from build123d import *

# Parameters (mm, degrees)
BOSS_EXTRUDE1_DEPTH = 25
SKETCH2_W           = 50
SKETCH2_H           = 35
SKETCH2_H_2         = 7.5
BOSS_EXTRUDE2_DEPTH = 100
SKETCH3_W           = 5
SKETCH3_H           = 7.5
BOSS_EXTRUDE3_DEPTH = 75
SKETCH4_W           = 10
SKETCH4_H           = 40
BOSS_EXTRUDE4_DEPTH = 7.5
CUT_EXTRUDE1_REACH  = 122.52
SKETCH5_W           = 30
SKETCH5_H           = 15
SKETCH7_W           = 42
SKETCH7_H           = 92
SKETCH7_W_2         = 38
SKETCH7_H_2         = 88
CUT_EXTRUDE2_DEPTH  = 15


with BuildPart() as part:
    # Sketch1 → Boss-Extrude1 (new, symmetric)
    with BuildSketch(Plane.XY):
        Polygon((0, 0), (45, 0), (0, 25), (-5, 25), (-5, 0), align=None)
    extrude(amount=BOSS_EXTRUDE1_DEPTH, both=True)

    # Sketch2 → Boss-Extrude2 (add)
    with BuildSketch(Plane(origin=(0, 0, 0), x_dir=(1, 0, 0), z_dir=(0, 1, 0))):
        with Locations((20, -7.5)):
            Rectangle(SKETCH2_W, SKETCH2_H)
        with Locations((20, 21.25)):
            Rectangle(SKETCH2_W, SKETCH2_H_2)
    extrude(amount=BOSS_EXTRUDE2_DEPTH)

    # Sketch3 → Boss-Extrude3 (add)
    with BuildSketch(Plane(origin=(0, 25, 0), x_dir=(1, 0, 0), z_dir=(0, 1, 0))):
        with Locations((-2.5, 13.75)):
            Rectangle(SKETCH3_W, SKETCH3_H)
    extrude(amount=BOSS_EXTRUDE3_DEPTH)

    # Sketch4 → Boss-Extrude4 (add)
    with BuildSketch(Plane.XY.offset(-17.5)):
        with Locations((40, 80)):
            Rectangle(SKETCH4_W, SKETCH4_H)
    extrude(amount=BOSS_EXTRUDE4_DEPTH)

    # Sketch5 → Cut-Extrude1 (cut, up to next)
    with BuildSketch(Plane.XY.offset(25), mode=Mode.PRIVATE) as cut_extrude1_sk1:
        with Locations((17.5, 77.5)):
            Rectangle(SKETCH5_W, SKETCH5_H)
    cut_extrude1_tool1 = extrude(cut_extrude1_sk1.sketch, amount=-CUT_EXTRUDE1_REACH, mode=Mode.PRIVATE) & part.part
    add(cut_extrude1_tool1.solids().sort_by_distance((17.5, 77.5, 25))[0], mode=Mode.SUBTRACT)

    # Sketch7 → Cut-Extrude2 (cut)
    with BuildSketch(Plane.XY.offset(25)):
        with Locations((20, 50)):
            Rectangle(SKETCH7_W, SKETCH7_H)
        with Locations((20, 50)):
            Rectangle(SKETCH7_W_2, SKETCH7_H_2, mode=Mode.SUBTRACT)
    extrude(amount=-CUT_EXTRUDE2_DEPTH, mode=Mode.SUBTRACT)


solid = part.part
CAD build for the part. Positions are in the model's coordinates, mm. A direction names the side the tool comes from. Give positions to 0.01 mm unless a question says otherwise; leave off trailing zeros. Loops run counter-clockwise (first coordinate to the right, second up) from the corner with the lowest first, then second, coordinate; pieces in that order, holes last. Notation, with made-up numbers: M -20,-19 L -6,-19 A8 ccw -6,-15 Z; hole C 64,-2 d4. An arc over 180 degrees is marked long. Answer in a Markdown table with one row per item. Add a question column.
Item 1: Probe probe 1 along X at (y, z) = (47.5, 12.5); probe 2 along Y at (x, z) = (18, 20); probe 3 along X at (y, z) = (83.5, 21). List the from-to ranges inside material, lowest first.
Item 2: Band-saw the part on B-B on y = 64. Give the cut face in (x, z).
Item 3: Drop flat-ended pins along their axis: P1, Ø1.5, axis at x = 7, z = -11.5, coming from the +Y side; P2, Ø2, axis at x = 8, y = 72, coming from the +Z side. Give the stop position or say it passes through.
Item 4: Band-saw the part on C-C on x = 31. Give the cut face in (y, z).
Item 5: Band-saw the part on D-D on z = -13. Give the cut face in (x, y).
Item 6: Mould opens along X. For faces 5 (the face through (40, 60, -14)), 6 (the face through (20, 4, 18)), 7 (the face through (-5, 49, 0)) say: +X half, -X half, draft (parallel to the pull), parting line (faces both ways), or undercut.
Item 7: Band-saw the part on A-A on z = 6. Give the cut face in (x, y).
Item 8: Tool access for faces 1 (the face through (20, 94, 18)), 2 (the face through (0, 62, -14)), 3 (the face through (22, 49, -17.5)), 4 (the face through (20, 51, -25)): list every direction of +Z, -Z, +X, -X, +Y, -Y with a clear straight run to the whole face (end or side of a thin tool).
Reply:
| question | item | result |
|---|---|---|
| 1 | probe 1 | x = -5 to -1, 1 to 39, 41 to 45 |
| 1 | probe 2 | y = 0 to 4, 6 to 70, 85 to 94, 96 to 100 |
| 1 | probe 3 | x = -5 to -1, 1 to 2.5, 32.5 to 39, 41 to 45 |
| 2 | outline | M -5,-25 L 45,-25 L 45,25 L 41,25 L 41,10 L 39,10 L 39,25 L 1,25 L 1,10 L -1,10 L -1,25 L -5,25 Z; hole M 0,-17.5 L 35,-17.5 L 35,-10 L 0,-10 Z |
| 3 | P1 | stops at y = 21.53 |
| 3 | P2 | stops at z = -17.5 |
| 4 | outline | M 0,-25 L 100,-25 L 100,-17.5 L 7.78,-17.5 L 7.78,-10 L 70,-10 L 70,25 L 6,25 L 6,10 L 4,10 L 4,25 L 0,25 Z; M 85,-10 L 100,-10 L 100,25 L 96,25 L 96,10 L 94,10 L 94,25 L 85,25 Z |
| 5 | outline | M -5,0 L 45,0 L 0,25 L 0,100 L -5,100 Z; M 35,60 L 45,60 L 45,100 L 35,100 Z |
| 6 | face 5 | draft |
| 6 | face 6 | undercut |
| 6 | face 7 | -X half |
| 7 | outline | M -5,0 L 45,0 L 45,100 L -5,100 Z; hole M 2.5,70 L 32.5,70 L 32.5,85 L 2.5,85 Z |
| 8 | face 1 | +Z |
| 8 | face 2 | +Y |
| 8 | face 3 | none |
| 8 | face 4 | -Z, +X, -X, +Y, -Y |
